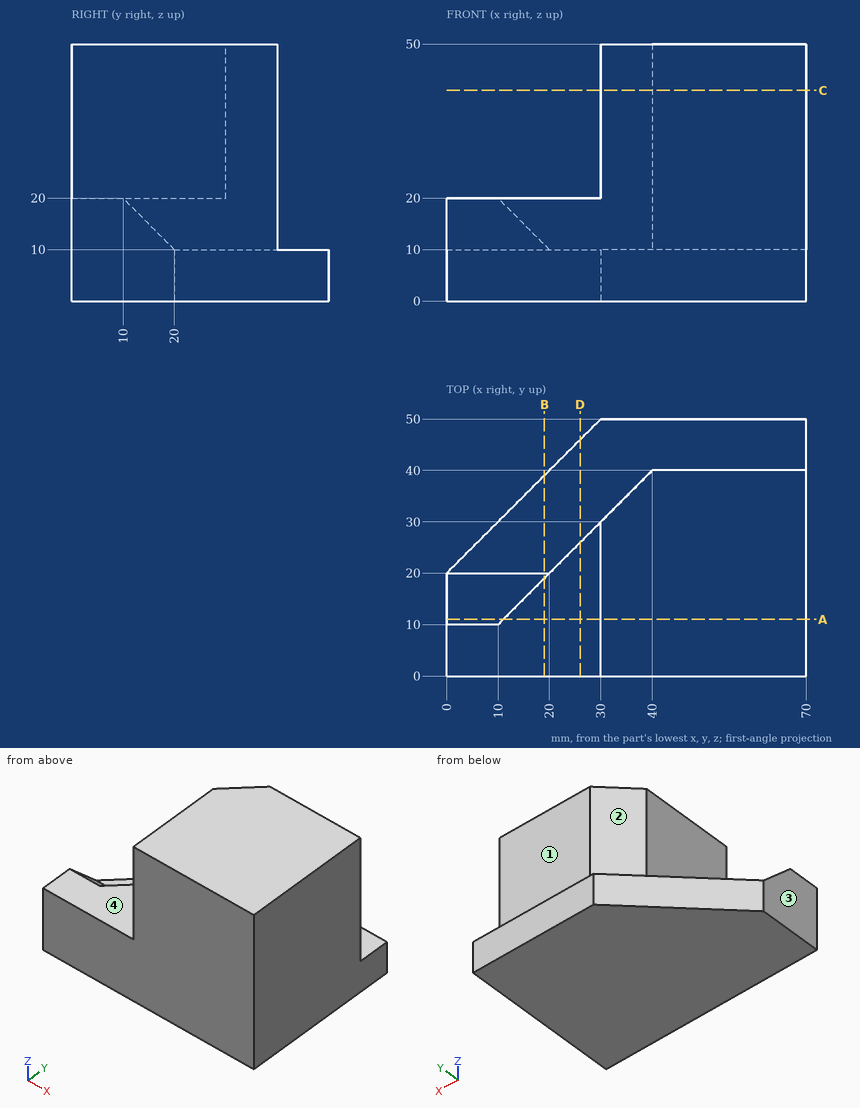
Check sheet for the drawn part. Datum: minimum x, y, z corner. Units: mm. A direction names the side the tool comes from. Give positions to 0.01 mm unless a question says otherwise; leave off trailing zeros. Order: outer loops, then holes, each group sorted by start corner. A loop starts at its lowest first (then second) coordinate and runs counter-clockwise, first axis right, second up. Notation, with made-up numbers: (33.5, 52) - (57.5, 52) arc R14 ccw to (57.5, 58) - close; hole circle Ø8 at (-0.75, 55.5). An arc over 180 degrees is marked (long way). Answer in a Markdown table with one row per item. Add a question column.
Q1. Gauge pin test, flat ends, axial feed: pin 1 (9 mm diameter, centred on x = 17.5, y = 12.5, fed in from +Z); pin 2 (5 mm diameter, centred on x = 24.5, y = 30.5, fed in from +Z); pin 3 (15 mm diameter, centred on y = 13, z = 28, fed in from -X). Record the tip position at first contact, or that the pin passes through.
Q2. Cross-section at C-C, the plane z = 41. Enter the section's corners in (x, y), then the cut area to 3 significant figures.
Q3. Cross-section at D-D, the plane x = 26. Enter the section's corners in (y, z).
Q4. Material ranges on probe 1 along Y at (x, z) = (20, 11); probe 2 along X at (y, z) = (14, 45.5); probe 3 along Z at (x, y) = (64, 41.5), recorded low to high. Write a range as from..to.
Q5. Cross-section at A-A, the plane y = 11. Enter the section's corners in (x, z), then the cut area to 3 significant figures.
Q6. Tool access check on the marked faces 1, 2, 3 and 4. Record the directions out of +Z, -Z, +X, -X, +Y, -Y that give a thin tool (end or side, any length) a straight path to the whole face; none if there is none.
Q7. Cross-section at B-B, the plane x = 19. Enter the section's corners in (y, z), then the cut area to 4 significant figures.
Check values:
| question | item | result |
|---|---|---|
| 1 | pin 1 | stops at z = 20 |
| 1 | pin 2 | stops at z = 10 |
| 1 | pin 3 | stops at x = 30 |
| 2 | outline | (30, 0) - (70, 0) - (70, 40) - (40, 40) - (30, 30) - close |
| 2 | area | 1,550 mm^2 |
| 3 | outline | (0, 0) - (46, 0) - (46, 10) - (26, 10) - (26, 20) - (0, 20) - close |
| 4 | probe 1 | y = 0..20 |
| 4 | probe 2 | x = 30..70 |
| 4 | probe 3 | z = 0..10 |
| 5 | outline | (0, 0) - (70, 0) - (70, 50) - (30, 50) - (30, 20) - (11, 20) - (11, 19) - (0, 19) - close |
| 5 | area | 2,590 mm^2 |
| 6 | face 1 | +Z, +X, -X, +Y |
| 6 | face 2 | +Z, -X, +Y |
| 6 | face 3 | +Z, -Z, -X, +Y, -Y |
| 6 | face 4 | +Z, -X, +Y, -Y |
| 7 | outline | (0, 0) - (39, 0) - (39, 10) - (20, 10) - (19, 11) - (19, 20) - (0, 20) - close |
| 7 | area | 580.5 mm^2 |
